```python
from build123d import *

# Parameters (mm, degrees)
F0_R     = 9.5
F0_R_2   = 7.75
F1_DEPTH = 3
F0_R_3   = 3.5
F2_DEPTH = 15
F0_R_4   = 1.75
F3_DEPTH = 5
F4_SIZE2 = 2.747477
F4_SIZE  = 1


with BuildPart() as f1:
    # F0 (on Top) → F1 (new body)
    with BuildSketch(Plane.XY):
        Circle(F0_R)
        Circle(F0_R_2, mode=Mode.SUBTRACT)
    extrude(amount=F1_DEPTH)

    # F0 (on Top) → F2 (join)
    with BuildSketch(Plane.XY):
        Circle(F0_R_2)
        Circle(F0_R_3, mode=Mode.SUBTRACT)
    extrude(amount=F2_DEPTH)

    # F0 (on Top) → F3 (join)
    with BuildSketch(Plane.XY):
        Circle(F0_R_3)
        Circle(F0_R_4, mode=Mode.SUBTRACT)
    extrude(amount=F3_DEPTH)

    # F4
    f4_edges = [f1.edges().sort_by_distance(p)[0] for p in [
        (-7.75, 0, 15),
    ]]
    chamfer(f4_edges, length=F4_SIZE, length2=F4_SIZE2)


solid = f1.part
```
For this review, take the finished solid that the model builds, in its own axes (mm). A direction names the side the tool comes from. Coordinates: 2 decimals unless noted, no trailing zeros. Order: outer loops, then holes, each group sorted by start corner. A loop starts at its lowest first (then second) coordinate and runs counter-clockwise, first axis right, second up. Notation, with made-up numbers: (72, -2.75) - (83, -2.75) arc R11 cw to (83, 7.25) - close; hole circle Ø9 at (5, -26.5). An arc over 180 degrees is marked (long way). Answer as a JSON object with one key per item and string values. Group by question number.
1. We need section A-A on y = 0. State the section outline as (x, z) points, then the cut area to 3 significant figures.
2. Clearance check with flat-ended pins moving along their axes: P1, Ø3.5, axis at x = 0, y = -1.5, coming from the +Z side; P2, Ø1, axis at y = -3, z = 6, coming from the -X side; P3, Ø8, axis at y = -4, z = 11, coming from the -X side. State where each tip first meets the part, or that it passes through.
3. The part is to be moulded in two halves that separate along Y. For faces 1 (the cylindrical face through (3.233, -1.341, 9.93)), 2 (the flat face through (-8, 0, 3)), 3 (the conical face through (3.144, -6.044, 14.828)), say which applies: pulls with the +Y half, pulls with the -Y half, needs draft (parallel to the pull), parting line crosses it, or undercut.
4. We need section D-D on z = 2.25. State the section outline as (x, y) points.
5. For faces 4 (the cylindrical face through (4.38, -8.43, 1.48)), 5 (the flat face through (-2, -1, 5)), list the 3-axis set-ups (+Z, -Z, +X, -X, +Y, -Y) from which the entire face can be reached by the end or side of a thin tool; tool diameter is ignored.
6. For probe 1 along Y at (x, z) = (0, 1.3); probe 2 along Y at (x, z) = (0, 11.5); probe 3 along Z at (x, y) = (-0.75, 2.25), list the stretches that pass through material, from the lowest coordinate up.
7. We need section C-C on z = 8.5. State the section outline as (x, y) points, then the cut area to 3 significant figures.
Final values:
{
 "1": {"outline": "(-9.5, 0) - (-1.75, 0) - (-1.75, 5) - (-3.5, 5) - (-3.5, 15) - (-6.75, 15) - (-7.75, 12.25) - (-7.75, 3) - (-9.5, 3) - close; (1.75, 0) - (9.5, 0) - (9.5, 3) - (7.75, 3) - (7.75, 12.25) - (6.75, 15) - (3.5, 15) - (3.5, 5) - (1.75, 5) - close", "area": "153 mm²"},
 "2": {"P1": "z = 5", "P2": "x = -7.34", "P3": "x = -7.75"},
 "3": {"face 1": "undercut", "face 2": "needs draft", "face 3": "parting line crosses it"},
 "4": {"outline": "circle Ø19 at (0, 0); hole circle Ø3.5 at (0, 0)"},
 "5": {"face 4": "+Z, -Z", "face 5": "+Z"},
 "6": {"probe 1": "-9.5 to -1.75, 1.75 to 9.5", "probe 2": "-7.75 to -3.5, 3.5 to 7.75", "probe 3": "0 to 5"},
 "7": {"outline": "circle Ø15.5 at (0, 0); hole circle Ø7 at (0, 0)", "area": "150 mm²"}
}
